Autodesk Inventor part; units mm, degrees
ref_plane "Work Plane1" through (12.5, 0, 0) normal (0, 0.5, 0.866) x (1, 0, 0)
ref_plane "YZ Plane" through (0, 0, 0) normal (1, 0, 0) x (0, 1, 0)
ref_plane "XZ Plane" through (0, 0, 0) normal (0, 1, 0) x (-1, 0, 0)
sketch "Sketch1" plane through (0, 0, 0) normal (0, 0, 1) x (1, 0, 0)
  line L0 (0, 0) -> (21.1667, 0)
  line L1 (25, 1.4434) -> (25, 2.5)
  line L2 (25, 2.5) -> (0, 2.5)
  line L3 (25, 1.4434) -> (22, 1.4434)
  line L4 (22, 1.4434) -> (21.1667, 0)
  line L5 (0, -0.5) -> (0, 3)
  line L6 (0, 2.5) -> (0, 0)
  dimension "d0" = 3
  dimension "d1" = 60
  dimension "d2" = 5
  dimension "d3" = 2.8868
  dimension "d5" = 25
revolve "Body" add sketch "Sketch1" angle 360 about axis through (0, 0, 0) along (1, 0, 0)
chamfer "Chamfer1" distance 0.4908 angle 45 1 edges at (25, -2.5, 0) measured on face at (25, 2.1236, -0.1994)
sketch "Sketch2" plane through (25, 0, 0) normal (1, 0, 0) x (0, 0, -1)
  circle A0 centre (0, 0) radius 1.4434
  line L0 (-0.7217, 1.25) -> (0.7217, 1.25)
  line L1 (0.7217, 1.25) -> (1.4434, 0)
  line L2 (1.4434, 0) -> (0.7217, -1.25)
  line L3 (0.7217, -1.25) -> (-0.7217, -1.25)
  line L4 (-0.7217, -1.25) -> (-1.4434, 0)
  line L5 (-1.4434, 0) -> (-0.7217, 1.25)
  point P0 (0, 0)
  point P1 (0, 0)
extrude "Slot" add sketch "Sketch2" against normal up to next contours L1 A0 | A0 L2 | L0 A0 | A0 L3 | L5 A0 | A0 L4
thread "Thread"
chamfer "Chamfer2" distance 0.4908 angle 45 1 edges at (0, -2.5, 0) measured on face at (8.1697, 2.4919, -0.2012)
ref_plane "Work Plane1" through (12.5, 0, 0) normal (0, 0.5, 0.866) x (1, 0, 0)
equation "\"d7\" = -0.5 * GD1 + 0.5 * NND"
equation "\"d8\" = FAWI"
equation "\"d29\" = -0.5 * GD1 + 0.5 * NND"
equation "\"d11\" = NLG"
equation "\"d13\" = -0.5 * GD1 + 0.5 * NND"
equation "\"d14\" = FAWI"
equation "\"d30\" = -0.5 * GD1 + 0.5 * NND"
equation "\"d0\" = INTI"
equation "\"d2\" = NND"
equation "\"d3\" = 1.1547 * SW"
equation "\"d5\" = NLG"
equation "\"NND\" = 5"
equation "\"NLG\" = 25"
equation "\"INTI\" = 3"
equation "\"FAWI\" = 45deg"
equation "\"SW\" = 2.5"
equation "\"GD1\" = THREADDIA - 1.2269 * PTC"
equation "\"FAWI1\" = 45deg"
equation "\"GUL\" = 0.61345 * PTC"
equation "\"SPD\" = 3.5"
equation "\"SEWI\" = 90deg"
equation "\"TOA\" = 30deg"
equation "\"THREADDIA\" = 5"
equation "\"PTC\" = 0.8"
equation "\"GAL\" = 0.61345 * PTC"
equation "\"E0\" = 1.155 * SW"
properties part number "DIN EN ISO 4026 - M5 x 25" material "Stainless Steel, 440C"
Build history of the part. All positions in model axes, mm. Give positions to 0.01 mm unless a question says otherwise; leave off trailing zeros. Order: outer loops, then holes, each group sorted by start corner. A loop starts at its lowest first (then second) coordinate and runs counter-clockwise, first axis right, second up. Notation, with made-up numbers: M -8,5.5 L 6,5.5 A27 ccw 6,26.5 Z; hole C 65.5,-11 d10. An arc over 180 degrees is marked long. Use one line per item in the form item = value.
1) Drop flat-ended pins along their axis: pin 1 (1 mm diameter, centred on x = 14.5, z = 1, fed in from -Y); pin 2 (1.5 mm diameter, centred on x = 3.5, z = 1, fed in from -Y); pin 3 (1.5 mm diameter, centred on x = 6, z = -1, fed in from +Y). Give the stop position or say it passes through.
Calculated:
pin_1 = -2.45
pin_2 = -2.49
pin_3 = 2.49
2) Two-plate mould, pull along Y, no slides. Class faces 1 (the face through (0, 0, 0)), 2 (the face through (23, 1.25, 0)), 3 (the face through (12.33, -0.54, 2.44)): released by +Y, released by -Y, zero draft, split by the parting line, or undercut.
Calculated:
face_1 = zero draft
face_2 = undercut
face_3 = split by the parting line
3) Saw through at A-A (x = 23.25). Give the cut face in (y, z), plus the area to 3 significant figures.
Calculated:
outline = C 0,0 d5; hole M -1.25,-0.72 L 0,-1.44 L 1.25,-0.72 L 1.25,0.72 L 0,1.44 L -1.25,0.72 Z
area = 14.2 mm2
4) Saw through at B-B (x = 13.5). Give the cut face in (y, z), plus the area to 3 significant figures.
Calculated:
outline = C 0,0 d5
area = 19.6 mm2
5) Probe probe 1 along Z at (x, y) = (19, 0.1); probe 2 along Z at (x, y) = (9, -1.55); probe 3 along Y at (x, z) = (12, 0.3). List the from-to ranges inside material, lowest first.
Calculated:
probe_1 = -2.5 to 2.5
probe_2 = -1.96 to 1.96
probe_3 = -2.48 to 2.48
